Here's how the part is built. I have some questions about the finished solid (model axes, mm). Face numbers are marked on the shaded views. A direction names the side the tool comes from. Coordinates: 2 decimals unless noted, no trailing zeros. Write each loop counter-clockwise with the first axis right and the second up, starting at its lowest first coordinate (ties: lowest second). Pieces come first, ordered by that corner, then holes.
(1) Imagine slicing it at D-D, the plane y = 3.25. List the corners of the cut face in (x, z) for me, plus the area to 3 significant figures.
(2) Imagine slicing it at B-B, the plane x = 0.7. List the corners of the cut face in (y, z) for me.
(3) For pin 1 Ø1.5 at (x, y) = (-1, 14) entering from -Z; pin 2 Ø1 at (x, y) = (1, 18) entering from -Z, each with a flat end and sliding along its axis, tell me the tip position at first contact or that it passes through.
(4) Which directions (+Z, -Z, +X, -X, +Y, -Y) give clear straight access to the entire face, cutting with the end or side of a thin tool? Please do the marked faces 1, 2 and 3.
(5) Imagine slicing it at A-A, the plane z = 0. List the corners of the cut face in (x, y) for me.
(6) Please list where these lines run through material, in increasing order: probe 1 along Y at (x, z) = (-0.25, -1.7); probe 2 along Z at (x, y) = (-0.05, 3); probe 3 along Z at (x, y) = (-0.15, 14.5).
(7) Imagine slicing it at C-C, the plane y = 18.5. List the corners of the cut face in (x, z) for me.
Autodesk Inventor part; units mm, degrees
ref_plane "YZ Plane" through (0, 0, 0) normal (1, 0, 0) x (0, 1, 0)
ref_plane "XZ Plane" through (0, 0, 0) normal (0, 1, 0) x (-1, 0, 0)
ref_plane "XY Plane" through (0, 0, 0) normal (0, 0, 1) x (1, 0, 0)
sketch "Sketch1" plane through (0, 0, 0) normal (0, 1, 0) x (-1, 0, 0)
  circle A0 centre (0, 0) radius 1.5
  dimension "d0" = 3
extrude "Extrusion1" add sketch "Sketch1" along normal blind 5
sketch "Sketch2" plane through (0, 5, 0) normal (0, 1, 0) x (1, 0, 0)
  circle A0 centre (0, 0) radius 1.5
  circle A1 centre (0, 0) radius 2.5
  line L0 (0, 2.5) -> (2.1651, 1.25)
  line L1 (2.1651, 1.25) -> (2.1651, -1.25)
  line L2 (2.1651, -1.25) -> (0, -2.5)
  line L3 (0, -2.5) -> (-2.1651, -1.25)
  line L4 (-2.1651, -1.25) -> (-2.1651, 1.25)
  line L5 (-2.1651, 1.25) -> (0, 2.5)
  dimension "d5" = 5
extrude "Extrusion2" add sketch "Sketch2" along normal blind 15 contours A0 | L1 L2 L3 L4 L5 L0
sketch "Sketch3" plane through (0, 20, 0) normal (0, 1, 0) x (1, 0, 0)
  circle A0 centre (0, 0) radius 1.5
  dimension "d8" = 3
extrude "Extrusion3" add sketch "Sketch3" along normal blind 5
thread "Thread1"
thread "Thread2"
properties part number "Heatbed_Standoff" material "Stainless Steel"
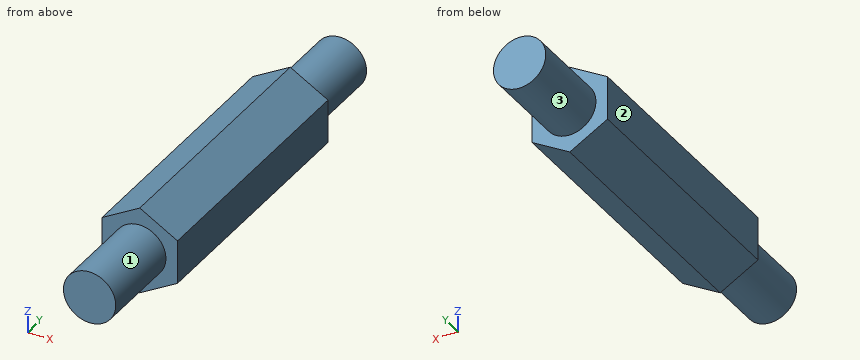
Recorded:
1. outline: circle Ø3 at (0, 0)
1. area: 7.07 mm2
2. outline: (0, -1.33) - (5, -1.33) - (5, -2.1) - (20, -2.1) - (20, -1.33) - (25, -1.33) - (25, 1.33) - (20, 1.33) - (20, 2.1) - (5, 2.1) - (5, 1.33) - (0, 1.33) - close
3. pin 1: stops at z = -2.36
3. pin 2: stops at z = -2.21
4. face 1: -Y
4. face 2: +Z, -Z, -X, +Y, -Y
4. face 3: +Y
5. outline: (-2.17, 5) - (-1.5, 5) - (-1.5, 0) - (1.5, 0) - (1.5, 5) - (2.17, 5) - (2.17, 20) - (1.5, 20) - (1.5, 25) - (-1.5, 25) - (-1.5, 20) - (-2.17, 20) - close
6. probe 1: y = 5 to 20
6. probe 2: z = -1.5 to 1.5
6. probe 3: z = -2.41 to 2.41
7. outline: (-2.17, -1.25) - (0, -2.5) - (2.17, -1.25) - (2.17, 1.25) - (0, 2.5) - (-2.17, 1.25) - close
